The listing builds one solid part. Answer for the finished solid, in the listing's coordinates (mm). Face numbers are marked on the shaded views. A direction names the side the tool comes from. Give positions to 0.01 mm unless a question says otherwise; leave off trailing zeros. Loops run counter-clockwise (first coordinate to the right, second up) from the corner with the lowest first, then second, coordinate; pieces in that order, holes last. Notation, with made-up numbers: (6.5, 79) - (39.5, 79) arc R28 cw to (39.5, 108) - close; hole circle Ø5 at (50.5, 30). An arc over 180 degrees is marked (long way). Write item = value, one per line. Start each with the question number.
1) The part is cut by section A-A on y = 0. Write down the section's boundary in (x, z), plus the area to 3 significant figures.
2) Flat-ended cylindrical pins translate along their axes: P1, Ø1.8, axis at y = 0, z = 0, coming from the +X side; P2, Ø0.8, axis at x = 0.5, y = 2, coming from the -Z side; P3, Ø4, axis at y = 1.5, z = -0.5, coming from the -X side. Find the tip coordinate at first contact, or state that the pin passes through.
3) Which of the six approach directions +Z, -Z, +X, -X, +Y, -Y give full straight-line access (tool end or side, diameter ignored) to the marked faces 1 and 2?
4) The part is cut by section C-C on x = 0.3. Write down the section's boundary in (y, z), plus the area to 3 significant figures.
5) The part is cut by section D-D on y = -0.75. Write down the section's boundary in (x, z), plus the area to 3 significant figures.
6) Consider probe 1 along Z at (x, y) = (0.35, 0); probe 2 along Z at (x, y) = (-0.4, 0); probe 3 along X at (y, z) = (-2.75, 1.25). Determine where each line is inside the solid, lowest interval first.
7) The part is cut by section B-B on z = 0. Write down the section's boundary in (x, y).
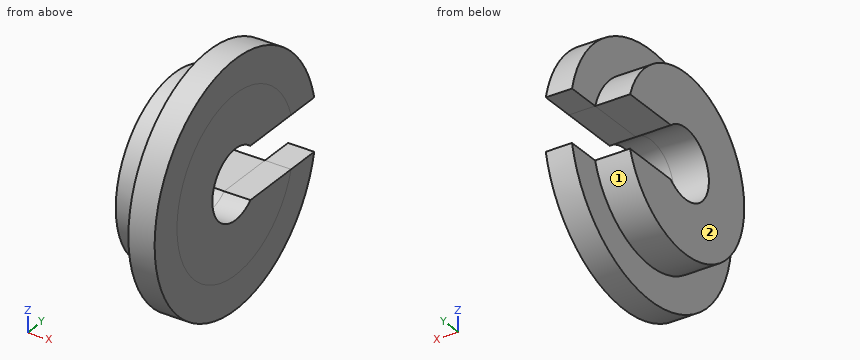
from build123d import *
from build123d.topology import SkipClean

# Parameters (mm, degrees)
BOSS_EXTRUDE1_DEPTH = 0.762
BOSS_EXTRUDE2_DEPTH = 1.778


with BuildPart() as part:
    # Sketch1 → Boss-Extrude1 (new body)
    with BuildSketch(Plane(origin=(0, 0, 0), x_dir=(0, 0, -1), z_dir=(1, 0, 0))):
        with BuildLine():
            Line((0.759321469, 3.430139815), (0.759321469, 0.655775721))
            ThreePointArc((0.759321469, 0.655775721), (0.004117603, -1.003291551), (-0.764678531, 0.649521081))
            Line((-0.764678531, 0.649521081), (-0.764678531, 3.428949546))
            ThreePointArc((-0.764678531, 3.428949546), (0.00274385, -3.51317815), (0.759321469, 3.430139815))
        make_face()
    extrude(amount=BOSS_EXTRUDE1_DEPTH)

    # Sketch3 → Boss-Extrude2 (add)
    with SkipClean():  # the faces are left unmerged after this step: merging them gives an invalid solid
        with BuildSketch(Plane(origin=(0.762, 0, 0), x_dir=(0, 0, -1), z_dir=(1, 0, 0))):
            with BuildLine():
                Line((-0.764678531, 2.423347628), (-0.764678531, 0.649521081))
                ThreePointArc((-0.764678531, 0.649521081), (0.004117603, -1.003291551), (0.759321469, 0.655775721))
                Line((0.759321469, 0.655775721), (0.759321469, 2.425031523))
                ThreePointArc((0.759321469, 2.425031523), (0.00280774, -2.541129493), (-0.764678531, 2.423347628))
            make_face()
        extrude(amount=-BOSS_EXTRUDE2_DEPTH)


solid = part.part
Answer below:
q1.outline = (-1.02, -2.54) - (0, -2.54) - (0, -3.51) - (0.76, -3.51) - (0.76, -1) - (-1.02, -1) - close; (-1.02, 1) - (0.76, 1) - (0.76, 3.51) - (0, 3.51) - (0, 2.54) - (-1.02, 2.54) - close
q1.area = 6.95 mm2
q2.P1 = through
q2.P2 = -3.13
q2.P3 = -1.02
q3.face_1 = -X
q3.face_2 = +Z, -Z, -X, +Y, -Y
q4.outline = (0.65, 0.76) - (3.43, 0.76) arc R3.51 ccw (long way) to (3.43, -0.76) - (0.66, -0.76) arc R1 cw (long way) to start
q4.area = 31.7 mm2
q5.outline = (-1.02, -2.43) - (0, -2.43) - (0, -3.43) - (0.76, -3.43) - (0.76, -0.67) - (-1.02, -0.67) - close; (-1.02, 0.67) - (0.76, 0.67) - (0.76, 3.43) - (0, 3.43) - (0, 2.43) - (-1.02, 2.43) - close
q5.area = 7.79 mm2
q6.probe_1 = -3.51 to -1, 1 to 3.51
q6.probe_2 = -2.54 to -1, 1 to 2.54
q6.probe_3 = 0 to 0.76
q7.outline = (-1.02, -2.54) - (0, -2.54) - (0, -3.51) - (0.76, -3.51) - (0.76, -1) - (-1.02, -1) - close
